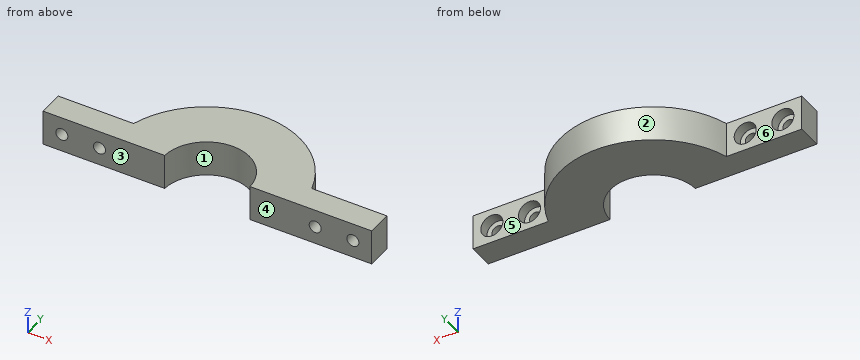
from build123d import *

# Parameters (mm, degrees)
BOSS_EXTRUDE1_DEPTH            = 7
CBORE_FOR_M2_SHCS1_D           = 2.4
CBORE_FOR_M2_SHCS1_CBORE_D     = 4.4
CBORE_FOR_M2_SHCS1_CBORE_DEPTH = 2


with BuildPart() as part:
    # Sketch1 → Boss-Extrude1 (new body)
    with BuildSketch(Plane.XY):
        with BuildLine():
            Line((-18.498310734, 0.25), (-32.739433475, 0.25))
            Line((-32.739433475, 0.25), (-32.739433475, 5.25))
            Line((-32.739433475, 5.25), (-17.739433475, 5.25))
            ThreePointArc((-17.739433475, 5.25), (0, 18.5), (17.739433475, 5.25))
            Line((17.739433475, 5.25), (32.739433475, 5.25))
            Line((32.739433475, 5.25), (32.739433475, 0.25))
            Line((32.739433475, 0.25), (18.498310734, 0.25))
            Line((18.498310734, 0.25), (8.496322734, 0.25))
            ThreePointArc((8.496322734, 0.25), (0, 8.5), (-8.496322734, 0.25))
            Line((-8.496322734, 0.25), (-18.498310734, 0.25))
        make_face()
    extrude(amount=-BOSS_EXTRUDE1_DEPTH)

    # CBORE for M2 SHCS1 (through all)
    with Locations(Plane(origin=(0, 5.25, 0), x_dir=(1, 0, 0), z_dir=(0, 1, 0))):
        with Locations((28.989433475, 3.5), (-28.989433475, 3.5), (-21.489433475, 3.5), (21.489433475, 3.5)):
            CounterBoreHole(CBORE_FOR_M2_SHCS1_D / 2, CBORE_FOR_M2_SHCS1_CBORE_D / 2, CBORE_FOR_M2_SHCS1_CBORE_DEPTH)


solid = part.part
Design review of the part built by this model. Coordinates are the model's own, in mm. Face numbers are marked on the shaded views. A direction names the side the tool comes from. Give positions to 0.01 mm unless a question says otherwise; leave off trailing zeros. Order: outer loops, then holes, each group sorted by start corner. A loop starts at its lowest first (then second) coordinate and runs counter-clockwise, first axis right, second up.
1. Mouldability with a two-part tool opening along X and no side actions: class the marked faces 1, 2 and 3 as +X half, -X half, draft (parallel to the pull), parting line (faces both ways), or undercut.
Solution:
face 1: undercut
face 2: parting line
face 3: draft
2. Add section A-A, the plane y = 7.5. State the section outline as (x, z) points.
Solution:
outline: (-16.91, -7) - (-4, -7) - (-4, 0) - (-16.91, 0) - close; (4, -7) - (16.91, -7) - (16.91, 0) - (4, 0) - close
3. For pin 1 Ø1.5 at (y, z) = (11, -3.5) entering from -X; pin 2 Ø3.5 at (x, z) = (-29.5, -3.5) entering from +Y; pin 3 Ø2 at (x, z) = (28.5, -3.5) entering from +Y, all flat-tipped, find the tip position at first contact; note any pin that passes through.
Solution:
pin 1: stops at x = -15.4
pin 2: stops at y = 5.25
pin 3: stops at y = 3.25
4. Add section C-C, the plane y = 10.75. State the section outline as (x, z) points.
Solution:
outline: (-15.06, -7) - (15.06, -7) - (15.06, 0) - (-15.06, 0) - close
5. Add section B-B, the plane x = 0. State the section outline as (y, z) points, then the cut area to 3 significant figures.
Solution:
outline: (8.5, -7) - (18.5, -7) - (18.5, 0) - (8.5, 0) - close
area: 70.0 mm2
6. To check wall thickness, follow L1, parallel to X at y = 6.5, z = -3.5; L2, parallel to Y at x = 19.5, z = -3.25; L3, parallel to Y at x = 0.5, z = -4.75. State the ranges of each line that lie inside material, in increasing order.
Solution:
L1: x = -17.32 to -5.48, 5.48 to 17.32
L2: y = 0.25 to 3.25
L3: y = 8.49 to 18.49
7. Tool access review of the marked faces 4, 5 and 6: name each direction out of +Z, -Z, +X, -X, +Y, -Y from which nothing blocks a thin tool from reaching the whole face with its end or side.
Solution:
face 4: +Z, -Z, +X, -X, -Y
face 5: +Z, -Z, +X, +Y
face 6: +Z, -Z, -X, +Y
